```python
from build123d import *

# Parameters (mm, degrees)
F0_W     = 40
F0_H     = 20
F1_DEPTH = 5
F2_R     = 6
F3_DEPTH = 10
F4_R     = 7
F5_DEPTH = 2
F6_R     = 7
F7_DEPTH = 2
F8_R     = 1.5
F9_R     = 0.99999


# Not quite as in the source:
# - a fillet or chamfer is up to 0.001 mm smaller than in the source, because OpenCascade refuses the exact size


with BuildPart() as f1:
    # F0 (on Top) → F1 (new body)
    with BuildSketch(Plane.XY):
        Rectangle(F0_W, F0_H)
    extrude(amount=F1_DEPTH)

    # F2 (on face) → F3 (join)
    with BuildSketch(Plane.XY.offset(5)):
        with Locations((-12, 0)):
            Circle(F2_R)
        with Locations((12, 0)):
            Circle(F2_R)
    extrude(amount=F3_DEPTH)

    # F4 (on face) → F5 (join)
    with BuildSketch(Plane.XY.offset(15)):
        with Locations((-12, 0)):
            Circle(F4_R)
    extrude(amount=F5_DEPTH)

    # F6 (on face) → F7 (join)
    with BuildSketch(Plane.XY.offset(15)):
        with Locations((12, 0)):
            Circle(F6_R)
    extrude(amount=F7_DEPTH)

    # F8
    f8_edges = [f1.edges().sort_by_distance(p)[0] for p in [
        (0, -10, 5),
        (-20, 0, 5),
        (0, 10, 5),
        (20, 0, 5),
        (20, -10, 2.5),
        (20, 10, 2.5),
        (-20, 10, 2.5),
        (-20, -10, 2.5),
    ]]
    fillet(f8_edges, radius=F8_R)

    # F9 (radius 1 in the source; OpenCascade refuses exactly that, so slightly less here)
    f9_edges = [f1.edges().sort_by_distance(p)[0] for p in [
        (-19, 0, 15),
        (5, 0, 15),
        (-19, 0, 17),
        (5, 0, 17),
    ]]
    fillet(f9_edges, radius=F9_R)


solid = f1.part
```
The listing builds one solid part. Answer for the finished solid, in the listing's coordinates (mm). A direction names the side the tool comes from. Coordinates: 2 decimals unless noted, no trailing zeros. Loops run counter-clockwise (first coordinate to the right, second up) from the corner with the lowest first, then second, coordinate; pieces in that order, holes last. Notation, with made-up numbers: (-16.5, 86) -> (4.5, 86) arc R28 ccw to (4.5, 118) -> close; hole circle Ø10 at (-7, 46.25). An arc over 180 degrees is marked (long way). Return JSON: item names as keys, results as strings. Group by question number.
(1) Determine the mould class of faces 1 (the cylindrical face through (17.54, -2.3, 9.93)), 2 (the flat face through (0, -10, 2)), 3 (the cylindrical face through (0.26, -9.55, 4.57)) for opening direction Z: released by +Z, released by -Z, zero draft, split by the parting line, or undercut.
(2) Find the intervals of material crossed by probe 1 along Z at (x, y) = (-8, -6); probe 2 along X at (y, z) = (-3.75, 11.25); probe 3 along X at (y, z) = (4.75, 10.5), in increasing order. Write a range as from..to.
(3) A cutting plane is placed at D-D on y = 8. Write down the section's boundary in (x, z).
(4) Given pin 1 Ø1 at (x, z) = (-14, 5) entering from -Y; pin 2 Ø2 at (x, y) = (-8, 6.5) entering from +Z; pin 3 Ø8.5 at (x, y) = (-2, -3) entering from +Z, each flat-ended and moving along its own axis, determine where each tip first touches the part or whether it passes through.
(5) Which of the six approach directions +Z, -Z, +X, -X, +Y, -Y give full straight-line access (tool end or side, diameter ignored) to faces 4 (the cylindrical face through (19.55, -9.57, 1.77)), 5 (the cylindrical face through (-6.277, 1.802, 9.93))?
(6) A cutting plane is placed at C-C on z = 14.5. Write down the section's boundary in (x, y).
The answers:
{
 "1": {"face 1": "undercut", "face 2": "zero draft", "face 3": "released by +Z"},
 "2": {"probe 1": "z = 0..5", "probe 2": "x = -16.68..-7.32, 7.32..16.68", "probe 3": "x = -15.67..-8.33, 8.33..15.67"},
 "3": {"outline": "(-20, 0) -> (20, 0) -> (20, 3.5) arc R1.5 ccw to (18.5, 5) -> (-18.5, 5) arc R1.5 ccw to (-20, 3.5) -> close"},
 "4": {"pin 1": "stops at y = -9.62", "pin 2": "stops at z = 16.77", "pin 3": "stops at z = 16.98"},
 "5": {"face 4": "+Z, -Z, +X, -Y", "face 5": "none"},
 "6": {"outline": "circle Ø12 at (-12, 0); circle Ø12 at (12, 0)"}
}
